Can you work these out from the model? Positions are in its coordinate system, mm. Face numbers are marked on the shaded views. A direction names the side the tool comes from. Give positions to 0.01 mm unless a question says otherwise; leave off trailing zeros. Write each loop counter-clockwise with the first axis right and the second up, starting at its lowest first coordinate (ties: lowest second). Pieces come first, ordered by that corner, then holes.
from build123d import *

# Parameters (mm, degrees)
SKETCH1_R           = 12.7
BOSS_EXTRUDE2_DEPTH = 50.8
CUT_EXTRUDE1_DEPTH  = 50.8
SKETCH3_R           = 2.54
BOSS_EXTRUDE3_DEPTH = 12.7
BOSS_EXTRUDE4_START = 12.7
SKETCH4_R           = 2.54
BOSS_EXTRUDE4_DEPTH = 12.7


with BuildPart() as part:
    # Sketch1 → Boss-Extrude2 (new body)
    with BuildSketch(Plane(origin=(0, 0, 0), x_dir=(1, 0, 0), z_dir=(0, 1, 0))):
        with Locations(Location((0, 0, 0), (0, 0, 270))):
            Circle(SKETCH1_R)
    extrude(amount=BOSS_EXTRUDE2_DEPTH)

    # Sketch2 → Cut-Extrude1 (cut)
    with BuildSketch(Plane(origin=(0, 50.8, 0), x_dir=(1, 0, 0), z_dir=(0, 1, 0))):
        Polygon((2.51878654, 10.627596076), (4.632126911, 12.867606004), (1.635551224, 13.577807488), align=None)
        Polygon((0, 10.922), (1.539793168, 13.589), (-1.539793168, 13.589), align=None)
        Polygon((4.901784646, 9.760255698), (7.474741494, 11.452516038), (4.722722626, 12.834631861), align=None)
        Polygon((7.020526273, 8.366737408), (9.914390828, 9.420017968), (7.555290828, 11.399537907), align=None)
        Polygon((8.760789511, 6.522166139), (11.819552786, 6.879684291), (9.980551347, 9.349891915), align=None)
        Polygon((10.028756319, 4.325983205), (13.087519594, 3.968465053), (11.867757759, 6.796190829), align=None)
        Polygon((10.756070278, 1.896585396), (13.649934833, 0.843304837), (13.115170278, 3.876105336), align=None)
        Polygon((10.903521705, -0.635057821), (13.476478552, -2.327318162), (13.655540573, 0.747058002), align=None)
        Polygon((10.463161454, -3.132464908), (12.576501825, -5.372474835), (13.459737141, -2.422263423), align=None)
        Polygon((9.45872946, -5.461), (10.998522628, -8.128), (12.538315796, -5.461), align=None)
        Polygon((7.944374913, -7.495131169), (8.82761023, -10.445342581), (10.940950601, -8.205332653), align=None)
        Polygon((6.001737058, -9.125197876), (6.180799079, -12.199574039), (8.753755927, -10.507313699), align=None)
        Polygon((3.735544005, -10.263322804), (3.20077945, -13.296123304), (6.094644005, -12.242842744), align=None)
        Polygon((1.267966808, -10.848149343), (0.048204973, -13.675875119), (3.106968247, -13.318356967), align=None)
        Polygon((-1.267966808, -10.848149343), (-3.106968247, -13.318356967), (-0.048204973, -13.675875119), align=None)
        Polygon((-3.735544005, -10.263322804), (-6.094644005, -12.242842744), (-3.20077945, -13.296123304), align=None)
        Polygon((-6.001737058, -9.125197876), (-8.753755927, -10.507313699), (-6.180799079, -12.199574039), align=None)
        Polygon((-7.944374913, -7.495131169), (-10.940950601, -8.205332653), (-8.82761023, -10.445342581), align=None)
        Polygon((-9.45872946, -5.461), (-12.538315796, -5.461), (-10.998522628, -8.128), align=None)
        Polygon((-10.463161454, -3.132464908), (-13.459737141, -2.422263423), (-12.576501825, -5.372474835), align=None)
        Polygon((-10.903521705, -0.635057821), (-13.655540573, 0.747058002), (-13.476478552, -2.327318162), align=None)
        Polygon((-10.756070278, 1.896585396), (-13.115170278, 3.876105336), (-13.649934833, 0.843304837), align=None)
        Polygon((-10.028756319, 4.325983205), (-11.867757759, 6.796190829), (-13.087519594, 3.968465053), align=None)
        Polygon((-8.760789511, 6.522166139), (-9.980551347, 9.349891915), (-11.819552786, 6.879684291), align=None)
        Polygon((-7.020526273, 8.366737408), (-7.555290828, 11.399537907), (-9.914390828, 9.420017968), align=None)
        Polygon((-4.901784646, 9.760255698), (-4.722722626, 12.834631861), (-7.474741494, 11.452516038), align=None)
        Polygon((-2.51878654, 10.627596076), (-1.635551224, 13.577807488), (-4.632126911, 12.867606004), align=None)
    extrude(amount=-CUT_EXTRUDE1_DEPTH, mode=Mode.SUBTRACT)

    # Sketch3 → Boss-Extrude3 (add)
    with BuildSketch(Plane(origin=(0, 0, 0), x_dir=(-1, 0, 0), z_dir=(0, -1, 0))):
        with Locations(Location((0, 0, 0), (0, 0, 270))):
            Circle(SKETCH3_R)
    extrude(amount=BOSS_EXTRUDE3_DEPTH)

    # Sketch4 → Boss-Extrude4 (add)
    with BuildSketch(Plane(origin=(0, 50.8, 0), x_dir=(1, 0, 0), z_dir=(0, 1, 0)).offset(BOSS_EXTRUDE4_START)):
        with Locations(Location((0, 0, 0), (0, 0, 270))):
            Circle(SKETCH4_R)
    extrude(amount=-BOSS_EXTRUDE4_DEPTH)


solid = part.part
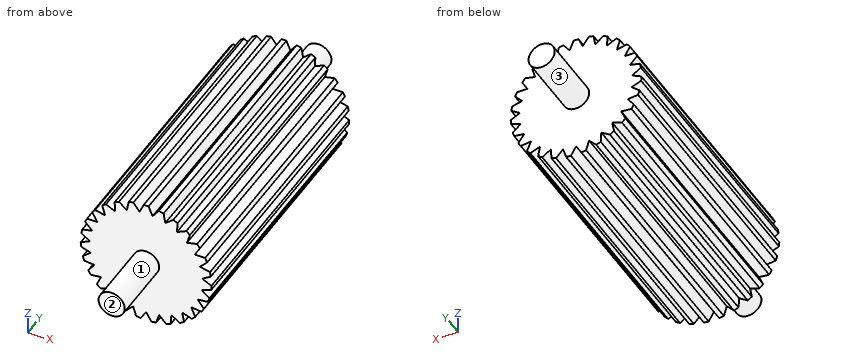
(1) Imagine slicing it at A-A, the plane y = -2.5. Write out the boundary of the cut face in (x, z), plus the area to 3 significant figures.
Returned:
outline: circle Ø5.08 at (0, 0)
area: 20.3 mm2
(2) For the marked faces 1, 2 and 3, which set-ups out of +Z, -Z, +X, -X, +Y, -Y let a thin tool reach every point of the face, with its end or its side?
Returned:
face 1: -Y
face 2: +Z, -Z, +X, -X, -Y
face 3: +Y
(3) Will these pins go through, and if not, where does the flat tip stop? P1, Ø10, axis at x = -8, z = 8, coming from the -Y side; P2, Ø1.6, axis at x = -11, y = 25, coming from the +Z side; P3, Ø10, axis at y = 54.5, z = -8, coming from the -X side.
Returned:
P1: stops at y = 0
P2: stops at z = 7.57
P3: stops at x = -11.23
(4) If I drill on L1, parallel to X at y = 48, z = -10.75; L2, parallel to Y at x = 2, z = -7.5; L3, parallel to X at y = 31, z = 1, over which ranges is the centre line in solid material (lowest first)?
Returned:
L1: x = -6.76 to -6.41, -4.84 to -2.63, -2.48 to 2.48, 2.63 to 4.84, 6.41 to 6.76
L2: y = 0 to 50.8
L3: x = -11.46 to 11.46
